```python
from build123d import *

# Parameters (mm, degrees)
SKETCH1_W                                      = 160
SKETCH1_H                                      = 60
BOSS_EXTRUDE1_DEPTH                            = 3
SKETCH2_R                                      = 1.1
SKETCH2_W                                      = 54
SKETCH2_H                                      = 37
CUT_EXTRUDE1_DEPTH                             = 171.906407136
FILLET1_R                                      = 2
FILLET2_R                                      = 3
CSK_FOR_M3_FLAT_HEAD_MACHINE_SCREW1_AT_2_COUNT = 2
CSK_FOR_M3_FLAT_HEAD_MACHINE_SCREW1_AT_2_PITCH = 22.5
CSK_FOR_M3_FLAT_HEAD_MACHINE_SCREW1_AT_3_COUNT = 2
CSK_FOR_M3_FLAT_HEAD_MACHINE_SCREW1_AT_3_PITCH = 45
CSK_FOR_M3_FLAT_HEAD_MACHINE_SCREW1_AT_4_COUNT = 2
CSK_FOR_M3_FLAT_HEAD_MACHINE_SCREW1_AT_4_PITCH = 79.056941504
CSK_FOR_M3_FLAT_HEAD_MACHINE_SCREW1_AT_5_COUNT = 2
CSK_FOR_M3_FLAT_HEAD_MACHINE_SCREW1_AT_5_PITCH = 65
CSK_FOR_M3_FLAT_HEAD_MACHINE_SCREW1_AT_6_COUNT = 2
CSK_FOR_M3_FLAT_HEAD_MACHINE_SCREW1_AT_6_PITCH = 130.000201211
CSK_FOR_M3_FLAT_HEAD_MACHINE_SCREW1_AT_7_COUNT = 2
CSK_FOR_M3_FLAT_HEAD_MACHINE_SCREW1_AT_7_PITCH = 131.97194743
CSK_FOR_M3_FLAT_HEAD_MACHINE_SCREW1_AT_8_COUNT = 2
CSK_FOR_M3_FLAT_HEAD_MACHINE_SCREW1_AT_8_PITCH = 137.493516675


with BuildPart() as part:
    # Sketch1 → Boss-Extrude1 (new body)
    with BuildSketch(Plane.XY):
        with Locations((80, 30)):
            Rectangle(SKETCH1_W, SKETCH1_H)
    extrude(amount=BOSS_EXTRUDE1_DEPTH)

    # Sketch2 → Cut-Extrude1 (cut, through all)
    with BuildSketch(Plane(origin=(0, 0, 0), x_dir=(-1, 0, 0), z_dir=(0, 0, -1))):
        with Locations((-109, 46.5)):
            Circle(SKETCH2_R)
        with Locations((-109, 18.5)):
            Circle(SKETCH2_R)
        with Locations((-51, 18.5)):
            Circle(SKETCH2_R)
        with Locations((-51, 46.5)):
            Circle(SKETCH2_R)
        with Locations((-80, 32.5)):
            Rectangle(SKETCH2_W, SKETCH2_H)
    extrude(amount=-CUT_EXTRUDE1_DEPTH, mode=Mode.SUBTRACT)

    # Fillet1
    fillet1_edges = [part.edges().sort_by_distance(p)[0] for p in [
        (160, 30, 0),
        (80, 0, 0),
        (0, 30, 0),
    ]]
    fillet(fillet1_edges, radius=FILLET1_R)

    # Fillet2
    # the kernel refuses this fillet: 3 mm, written as the material it takes off along each edge
    with BuildSketch(Plane(origin=(3, 3, 0), x_dir=(0, -1, 0), z_dir=(1, 0, 0))) as fillet2_piece_1:
        with BuildLine():
            CenterArc((1, -2), 2, 0, 90)
            Line((3, -2), (3, 0))
            Line((3, 0), (1, 0))
        make_face()
    revolve(axis=Axis((3, 3, 0), (0, 0, -1)), revolution_arc=90, mode=Mode.SUBTRACT)
    with BuildSketch(Plane(origin=(157, 3, 0), x_dir=(1, 0, 0), z_dir=(0, 1, 0))) as fillet2_piece_2:
        with BuildLine():
            CenterArc((1, -2), 2, 0, 90)
            Line((3, -2), (3, 0))
            Line((3, 0), (1, 0))
        make_face()
    revolve(axis=Axis((157, 3, 0), (0, 0, -1)), revolution_arc=90, mode=Mode.SUBTRACT)
    with BuildSketch(Plane(origin=(160, 0, 0), x_dir=(-1, 0, 0), z_dir=(0, 0, 1))) as fillet2_piece_3:
        with BuildLine():
            CenterArc((FILLET2_R, -FILLET2_R), FILLET2_R, 90, 90)
            Line((0, -FILLET2_R), (0, 0))
            Line((0, 0), (FILLET2_R, 0))
        make_face()
    extrude(amount=10.5, mode=Mode.SUBTRACT)
    with BuildSketch(Plane(origin=(0, 0, 0), x_dir=(1, 0, 0), z_dir=(0, 0, 1))) as fillet2_piece_4:
        with BuildLine():
            CenterArc((FILLET2_R, FILLET2_R), FILLET2_R, 180, 90)
            Line((0, FILLET2_R), (0, 0))
            Line((0, 0), (FILLET2_R, 0))
        make_face()
    extrude(amount=10.5, mode=Mode.SUBTRACT)

    # Sketch5 → CSK for M3 Flat Head Machine Screw1 (revolve, cut)
    with BuildSketch(Plane(origin=(145, 55, 0), x_dir=(0, 1, 0), z_dir=(1, 0, 0))):
        Polygon((0, 0), (0, 3), (1.7, 3), (1.7, 1.45), (3.15, 0), align=None)
    csk_for_m3_flat_head_machine_screw1 = revolve(axis=Axis((145, 55, -6.35), (0, 0, 1)), mode=Mode.SUBTRACT)

    # CSK for M3 Flat Head Machine Screw1 at 2: CSK for M3 Flat Head Machine Screw1 ×2
    with Locations(*[(0, -i * CSK_FOR_M3_FLAT_HEAD_MACHINE_SCREW1_AT_2_PITCH, 0) for i in range(1, CSK_FOR_M3_FLAT_HEAD_MACHINE_SCREW1_AT_2_COUNT)]):
        add(csk_for_m3_flat_head_machine_screw1, mode=Mode.SUBTRACT)

    # CSK for M3 Flat Head Machine Screw1 at 3: CSK for M3 Flat Head Machine Screw1 ×2
    with Locations(*[(0, -i * CSK_FOR_M3_FLAT_HEAD_MACHINE_SCREW1_AT_3_PITCH, 0) for i in range(1, CSK_FOR_M3_FLAT_HEAD_MACHINE_SCREW1_AT_3_COUNT)]):
        add(csk_for_m3_flat_head_machine_screw1, mode=Mode.SUBTRACT)

    # CSK for M3 Flat Head Machine Screw1 at 4: CSK for M3 Flat Head Machine Screw1 ×2
    with Locations(*[Vector(-0.8221921916437787, -0.5692099788303083, 0) * (i * CSK_FOR_M3_FLAT_HEAD_MACHINE_SCREW1_AT_4_PITCH) for i in range(1, CSK_FOR_M3_FLAT_HEAD_MACHINE_SCREW1_AT_4_COUNT)]):
        add(csk_for_m3_flat_head_machine_screw1, mode=Mode.SUBTRACT)

    # CSK for M3 Flat Head Machine Screw1 at 5: CSK for M3 Flat Head Machine Screw1 ×2
    with Locations(*[(-i * CSK_FOR_M3_FLAT_HEAD_MACHINE_SCREW1_AT_5_PITCH, 0, 0) for i in range(1, CSK_FOR_M3_FLAT_HEAD_MACHINE_SCREW1_AT_5_COUNT)]):
        add(csk_for_m3_flat_head_machine_screw1, mode=Mode.SUBTRACT)

    # CSK for M3 Flat Head Machine Screw1 at 6: CSK for M3 Flat Head Machine Screw1 ×2
    with Locations(*[Vector(-0.9999984522282437, 0.0017594149928170457, 0) * (i * CSK_FOR_M3_FLAT_HEAD_MACHINE_SCREW1_AT_6_PITCH) for i in range(1, CSK_FOR_M3_FLAT_HEAD_MACHINE_SCREW1_AT_6_COUNT)]):
        add(csk_for_m3_flat_head_machine_screw1, mode=Mode.SUBTRACT)

    # CSK for M3 Flat Head Machine Screw1 at 7: CSK for M3 Flat Head Machine Screw1 ×2
    with Locations(*[Vector(-0.9850578288164882, -0.17222390625968964, 0) * (i * CSK_FOR_M3_FLAT_HEAD_MACHINE_SCREW1_AT_7_PITCH) for i in range(1, CSK_FOR_M3_FLAT_HEAD_MACHINE_SCREW1_AT_7_COUNT)]):
        add(csk_for_m3_flat_head_machine_screw1, mode=Mode.SUBTRACT)

    # CSK for M3 Flat Head Machine Screw1 at 8: CSK for M3 Flat Head Machine Screw1 ×2
    with Locations(*[Vector(-0.9454991271168818, -0.3256246314719061, 0) * (i * CSK_FOR_M3_FLAT_HEAD_MACHINE_SCREW1_AT_8_PITCH) for i in range(1, CSK_FOR_M3_FLAT_HEAD_MACHINE_SCREW1_AT_8_COUNT)]):
        add(csk_for_m3_flat_head_machine_screw1, mode=Mode.SUBTRACT)


solid = part.part
```
Work out the finished part from the listing and answer in its coordinate system (mm). A direction names the side the tool comes from. Give positions to 0.01 mm unless a question says otherwise; leave off trailing zeros. Loops run counter-clockwise (first coordinate to the right, second up) from the corner with the lowest first, then second, coordinate; pieces in that order, holes last. Notation, with made-up numbers: (22, -26) -> (41, -26) arc R13 ccw to (41, -8) -> close; hole circle Ø1 at (51, 84). An arc over 180 degrees is marked (long way). Use CSV: the item, a comma, the result in double quotes.
1. Straight lines are drawn through the part: line 1 (X direction, y = 10, z = 2.1); line 2 (Y direction, x = 15, z = 1.9); line 3 (Y direction, x = 58, z = 2.5). For each, find the intervals that lie inside material, in ascending order.
Found:
line 1,"0 to 13.32, 16.68 to 78.3, 81.7 to 143.3, 146.7 to 160"
line 2,"0 to 8.53, 11.93 to 30.57, 33.97 to 53.53, 56.93 to 60"
line 3,"0 to 14, 51 to 60"
2. The part is cut by section B-B (x = 68.5). Write down the section's boundary in (y, z).
Found:
outline,"(0, 2) arc R2 ccw to (2, 0) -> (14, 0) -> (14, 3) -> (0, 3) -> close; (51, 0) -> (60, 0) -> (60, 3) -> (51, 3) -> close"
3. A tool of negligible diameter and unlimited length cuts with its end or side. For faces 1 (the cylindrical face through (0.86, 0.9, 2.49)), 2 (the flat face through (107, 32, 1)), from which of +Z, -Z, +X, -X, +Y, -Y can it reach the whole face along a straight path? Write none if from no direction.
Found:
face 1,"+Z, -Z, -X, -Y"
face 2,"+Z, -Z"
4. The part is cut by section A-A (x = 15). Write down the section's boundary in (y, z), then the cut area to 3 significant figures.
Found:
outline,"(0, 2) arc R2 ccw to (2, 0) -> (7.08, 0) -> (8.53, 1.45) -> (8.53, 3) -> (0, 3) -> close; (11.93, 1.45) -> (13.38, 0) -> (29.12, 0) -> (30.57, 1.45) -> (30.57, 3) -> (11.93, 3) -> close; (33.97, 1.45) -> (35.42, 0) -> (52.08, 0) -> (53.53, 1.45) -> (53.53, 3) -> (33.97, 3) -> close; (56.93, 1.45) -> (58.38, 0) -> (60, 0) -> (60, 3) -> (56.93, 3) -> close"
area,"142 mm^2"
5. Flat-ended cylindrical pins translate along their axes: pin 1 Ø1.3 at (x, y) = (51, 46.5) entering from -Z; pin 2 Ø5.5 at (x, y) = (15, 10.23) entering from -Z; pin 3 Ø1.5 at (y, z) = (13.5, 1) entering from +X; pin 4 Ø4 at (x, y) = (145, 55) entering from +Z. Find the tip coordinate at first contact, or state that the pin passes through.
Found:
pin 1,"through"
pin 2,"z = 0.4"
pin 3,"x = 159.98"
pin 4,"z = 3"
6. The part is cut by section C-C (y = 55). State how many separate pieces and enclosed holes the cut face has, then the cut area to 3 significant figures.
Found:
separate pieces,"4"
enclosed holes,"0"
area,"441 mm^2"
7. The mould has two halves that part along Y. Classify faces 3 (the flat face through (79, 60, 1)), 4 (the flat face through (79, 6, 0)), 5 (the flat face through (80, 14, 1)), 6 (the cylindrical face through (159.1, 0.86, 2.49)): +Y half, -Y half, draft (parallel to the pull), parting line (faces both ways), or undercut.
Found:
face 3,"+Y half"
face 4,"draft"
face 5,"undercut"
face 6,"-Y half"
